Could you check a few things on this model? Use its own coordinates, in mm. Face numbers are marked on the shaded views. A direction names the side the tool comes from. Round coordinates to 2 decimals unless told otherwise and drop trailing zeros. Write each loop counter-clockwise with the first axis right and the second up, starting at its lowest first coordinate (ties: lowest second). Pieces come first, ordered by that corner, then holes. Notation, with made-up numbers: M 85,53 L 94,53 A23 cw 94,71 Z; hole C 41,-34.75 d5. An arc over 180 degrees is marked long. One line per item, written item: value. Start each with the question number.
(1) Thinking about a two-plate mould opening in X: for the marked faces 1, 2 and 3, which applies, released by +X, released by -X, zero draft, split by the parting line, or undercut?
(2) I want a section at D-D on y = -4. Please give me the cut outline in (x, z), and give its area (3 significant figures).
(3) If I drill on L1, parallel to X at y = -3.75, z = -4.75; L2, parallel to Y at x = -32.75, z = -5.9; L3, parallel to X at y = -0.75, z = -1.75, over which ranges is the centre line in solid material (lowest first)?
(4) I'm going to push flat-ended pins straight in: pin 1 Ø2 at (y, z) = (-3.5, -1) entering from +X; pin 2 Ø1 at (x, y) = (-10, 1) entering from -Z; pin 3 Ø3.5 at (y, z) = (-1, -2) entering from -X. Where does each tip first touch, or does it pass through?
(5) I want a section at A-A on z = -2.75. Please give me the cut outline in (x, y).
(6) I want a section at B-B on y = 2.75. Please give me the cut outline in (x, z), and give its area (3 significant figures).
(7) I want a section at C-C on x = -32.75. Please give me the cut outline in (y, z).
(8) Which directions (+Z, -Z, +X, -X, +Y, -Y) give clear straight access to the entire face, cutting with the end or side of a thin tool? Please do the marked faces 4, 5, 6 and 7.
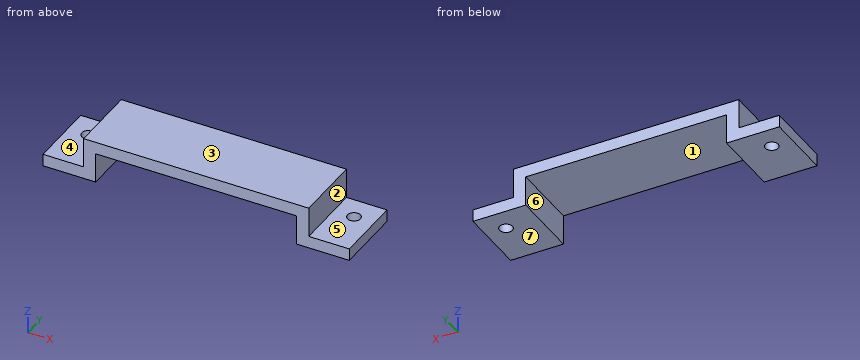
```python
from build123d import *

# Parameters (mm, degrees)
ESBO_O1_W                = 55.5
ESBO_O1_H                = 17
RESSALTO_EXTRUS_O1_DEPTH = 3
ESBO_O9_W                = 3
ESBO_O9_H                = 17
RESSALTO_EXTRUS_O5_DEPTH = 7.4
ESBO_O10_W               = 10
ESBO_O10_H               = 3
RESSALTO_EXTRUS_O6_DEPTH = 17
CORTE_EXTRUS_O4_REACH    = 41.396
ESBO_O11_R               = 1.6


with BuildPart() as part:
    # Esboço1 → Ressalto-extrusão1 (new body)
    with BuildSketch(Plane.XY):
        Rectangle(ESBO_O1_W, ESBO_O1_H)
    extrude(amount=RESSALTO_EXTRUS_O1_DEPTH)

    # Esboço9 → Ressalto-extrusão5 (add)
    with BuildSketch(Plane(origin=(0, 0, 0), x_dir=(-1, 0, 0), z_dir=(0, 0, -1))):
        with Locations((-26.25, 0)):
            Rectangle(ESBO_O9_W, ESBO_O9_H)
        with Locations((26.25, 0)):
            Rectangle(ESBO_O9_W, ESBO_O9_H)
    extrude(amount=RESSALTO_EXTRUS_O5_DEPTH)

    # Esboço10 → Ressalto-extrusão6 (add, through all)
    with BuildSketch(Plane(origin=(0, 8.5, 0), x_dir=(1, 0, 0), z_dir=(0, 1, 0))):
        with Locations((32.75, 5.9)):
            Rectangle(ESBO_O10_W, ESBO_O10_H)
        with Locations((-32.75, 5.9)):
            Rectangle(ESBO_O10_W, ESBO_O10_H)
    extrude(amount=-RESSALTO_EXTRUS_O6_DEPTH)

    # Esboço11 → Corte-extrusão4 (cut, up to next)
    with BuildSketch(Plane.XY.offset(-4.4), mode=Mode.PRIVATE) as corte_extrus_o4_sk1:
        with Locations((-32.75, 2.75)):
            Circle(ESBO_O11_R)
    corte_extrus_o4_tool1 = extrude(corte_extrus_o4_sk1.sketch, amount=-CORTE_EXTRUS_O4_REACH, mode=Mode.PRIVATE) & part.part
    # Esboço11 → Corte-extrusão4 (cut, up to next)
    with BuildSketch(Plane.XY.offset(-4.4), mode=Mode.PRIVATE) as corte_extrus_o4_sk2:
        with Locations(Location((32.75, 2.75, 0), (0, 0, 180))):
            Circle(ESBO_O11_R)
    corte_extrus_o4_tool2 = extrude(corte_extrus_o4_sk2.sketch, amount=-CORTE_EXTRUS_O4_REACH, mode=Mode.PRIVATE) & part.part
    add(corte_extrus_o4_tool1.solids().sort_by_distance((-32.75, 2.75, -4.4))[0], mode=Mode.SUBTRACT)
    add(corte_extrus_o4_tool2.solids().sort_by_distance((32.75, 2.75, -4.4))[0], mode=Mode.SUBTRACT)


solid = part.part
```
Found:
1. face 1: undercut
1. face 2: released by +X
1. face 3: zero draft
2. outline: M -37.75,-7.4 L -24.75,-7.4 L -24.75,0 L 24.75,0 L 24.75,-7.4 L 37.75,-7.4 L 37.75,-4.4 L 27.75,-4.4 L 27.75,3 L -27.75,3 L -27.75,-4.4 L -37.75,-4.4 Z
2. area: 271 mm²
3. L1: x = -37.75 to -24.75, 24.75 to 37.75
3. L2: y = -8.5 to 1.15, 4.35 to 8.5
3. L3: x = -27.75 to -24.75, 24.75 to 27.75
4. pin 1: stops at x = 27.75
4. pin 2: stops at z = 0
4. pin 3: stops at x = -27.75
5. outline: M -27.75,-8.5 L -24.75,-8.5 L -24.75,8.5 L -27.75,8.5 Z; M 24.75,-8.5 L 27.75,-8.5 L 27.75,8.5 L 24.75,8.5 Z
6. outline: M -37.75,-7.4 L -34.35,-7.4 L -34.35,-4.4 L -37.75,-4.4 Z; M -31.15,-7.4 L -24.75,-7.4 L -24.75,0 L 24.75,0 L 24.75,-7.4 L 31.15,-7.4 L 31.15,-4.4 L 27.75,-4.4 L 27.75,3 L -27.75,3 L -27.75,-4.4 L -31.15,-4.4 Z; M 34.35,-7.4 L 37.75,-7.4 L 37.75,-4.4 L 34.35,-4.4 Z
6. area: 252 mm²
7. outline: M -8.5,-7.4 L 1.15,-7.4 L 1.15,-4.4 L -8.5,-4.4 Z; M 4.35,-7.4 L 8.5,-7.4 L 8.5,-4.4 L 4.35,-4.4 Z
8. face 4: +Z, -X, +Y, -Y
8. face 5: +Z, +X, +Y, -Y
8. face 6: -Z, +Y, -Y
8. face 7: -Z, +X, -X, +Y, -Y
